from build123d import *

# Parameters (mm, degrees)
BOSS_EXTRU_1_DEPTH = 5.125
ESQUISSE2_R        = 2.5
BOSS_EXTRU_2_DEPTH = 10
ESQUISSE3_R        = 4
BOSS_EXTRU_3_DEPTH = 15


with BuildPart() as part:
    # Esquisse1 → Boss.-Extru.1 (new, symmetric)
    with BuildSketch(Plane.XY):
        with BuildLine():
            Line((-28.790189362, 6.603053435), (145.209810638, 6.603053435))
            ThreePointArc((145.209810638, 6.603053435), (150.209810638, 1.603053435), (145.209810638, -3.396946565))
            Line((145.209810638, -3.396946565), (-28.790189362, -3.396946565))
            ThreePointArc((-28.790189362, -3.396946565), (-33.790189362, 1.603053435), (-28.790189362, 6.603053435))
        make_face()
    extrude(amount=BOSS_EXTRU_1_DEPTH, both=True)

    # Esquisse2 → Boss.-Extru.2 (add)
    with BuildSketch(Plane.XY):
        with Locations((-28.790189362, 1.603053435)):
            Circle(ESQUISSE2_R)
    extrude(amount=BOSS_EXTRU_2_DEPTH)

    # Esquisse3 → Boss.-Extru.3 (add)
    with BuildSketch(Plane.XY):
        with Locations((145.209810638, 1.603053435)):
            Circle(ESQUISSE3_R)
    extrude(amount=-BOSS_EXTRU_3_DEPTH)


solid = part.part
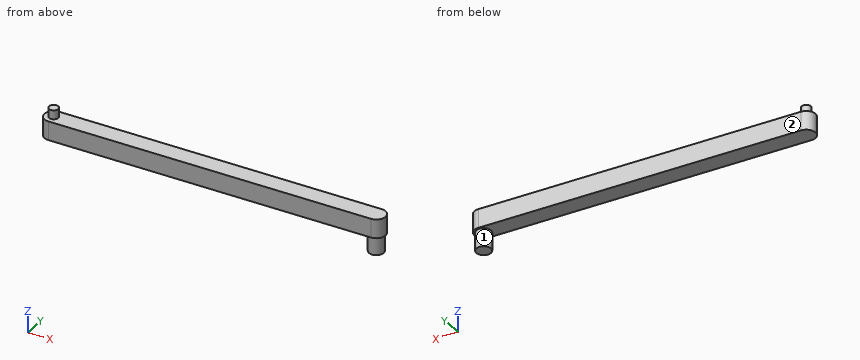
Design review of the part built by this model. Coordinates are the model's own, in mm. Face numbers are marked on the shaded views. A direction names the side the tool comes from. Give positions to 0.01 mm unless a question says otherwise; leave off trailing zeros. Write each loop counter-clockwise with the first axis right and the second up, starting at its lowest first coordinate (ties: lowest second). Pieces come first, ordered by that corner, then holes. Notation, with made-up numbers: M 86,6.5 L 136,6.5 A29 ccw 136,36.5 Z; hole C -24.5,62 d4. An arc over 180 degrees is marked long. Return JSON: item names as keys, results as strings. Group by question number.
Item 1: Wall thickness on line 1 along Z through (x, y) = (113.5, 0) (3 decimals); line 2 along X through (y, z) = (1.25, -8); line 3 along X through (y, z) = (-2.25, -3.75): over which ranges is each line inside the solid? List them lowest first.
Item 2: Tool access review of the marked faces 1 and 2: name each direction out of +Z, -Z, +X, -X, +Y, -Y from which nothing blocks a thin tool from reaching the whole face with its end or side.
Item 3: Take a section at B-B (z = -11.5). Give the boundary of the cut face in (x, y).
Item 4: Clearance check with flat-ended pins moving along their axes: pin 1 Ø5 at (x, y) = (59.5, 2) entering from +Z (3 decimals); pin 2 Ø5 at (x, y) = (127, -2) entering from -Z (3 decimals); pin 3 Ø1.5 at (y, z) = (-0.5, -12) entering from +X. State where each tip first meets the part, or that it passes through.
Item 5: Take a section at A-A (x = 118.5). Give the boundary of the cut face in (y, z) (3 decimals).
Return value:
{
 "1": {"line 1": "z = -5.125 to 5.125", "line 2": "x = 141.23 to 149.19", "line 3": "x = -31.98 to 148.4"},
 "2": {"face 1": "-Z", "face 2": "+Z, -Z, +X, -X, +Y"},
 "3": {"outline": "C 145.21,1.6 d8"},
 "4": {"pin 1": "stops at z = 5.125", "pin 2": "stops at z = -5.125", "pin 3": "stops at x = 148.97"},
 "5": {"outline": "M -3.397,-5.125 L 6.603,-5.125 L 6.603,5.125 L -3.397,5.125 Z"}
}
